```python
from build123d import *

# Parameters (mm, degrees)
BOSS_EXTRUDE1_DEPTH = 7.5
FILLET1_R           = 0.4
SKETCH3_R           = 3
CUT_EXTRUDE2_DEPTH  = 1


with BuildPart() as part:
    # Sketch1 → Boss-Extrude1 (new body)
    with BuildSketch(Plane.XY):
        Polygon((9.332731301, -89.971589642), (0, -80.638858341), (-9.332731301, -89.971589642), align=None)
    extrude(amount=-BOSS_EXTRUDE1_DEPTH)

    # Sketch2 → section 1 of loft1
    with BuildSketch(Plane.XY.offset(1.5875), mode=Mode.PRIVATE) as loft1_s1:
        Polygon((-13.165295331, -91.559089642), (13.165295331, -91.559089642), (0, -78.393794311), align=None)
    # loft from a face of the part (loft1)
    loft([part.faces().sort_by_distance((0, -86.860679209, 0))[0], loft1_s1.sketch])

    # Fillet1
    fillet1_edges = [part.edges().sort_by_distance(p)[0] for p in [
        (-4.666365651, -85.305223992, -7.5),
        (0, -89.971589642, -7.5),
        (4.666365651, -85.305223992, -7.5),
    ]]
    fillet(fillet1_edges, radius=FILLET1_R)

    # Sketch3 → Cut-Extrude2 (cut)
    with BuildSketch(Plane.XY.offset(1.5875)):
        with Locations((0, -86.105845763)):
            Circle(SKETCH3_R)
    extrude(amount=-CUT_EXTRUDE2_DEPTH, mode=Mode.SUBTRACT)


solid = part.part
```
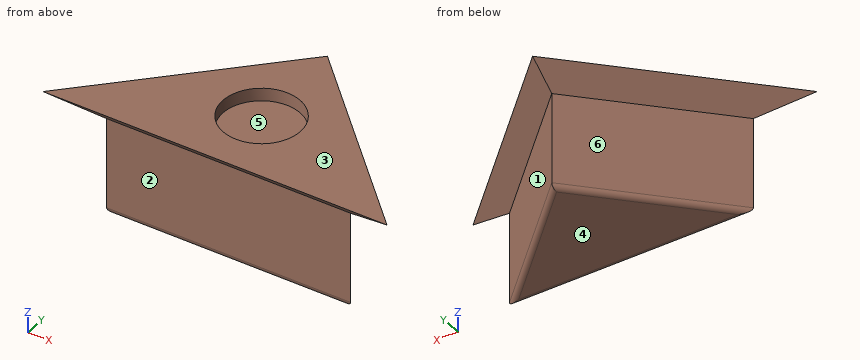
The listing builds one solid part. Answer for the finished solid, in the listing's coordinates (mm). Face numbers are marked on the shaded views. A direction names the side the tool comes from. Coordinates: 2 decimals unless noted, no trailing zeros. Order: outer loops, then holes, each group sorted by start corner. A loop starts at its lowest first (then second) coordinate and runs counter-clockwise, first axis right, second up. Notation, with made-up numbers: M -23.5,-10.75 L 25.5,-10.75 A15 ccw 25.5,4.25 Z; hole C 69.25,89 d1. An arc over 180 degrees is marked long. Answer as a JSON object with one key per item and string values. Group by question number.
1. Section A-A on z = -1 is taken. Write down the section's boundary in (x, y).
2. Flat-ended cylindrical pins translate along their axes: P1, Ø1.5, axis at x = -10.5, z = 0.5, coming from the -Y side; P2, Ø1, axis at x = -2, z = -6, coming from the -Y side; P3, Ø2, axis at y = -80.5, z = -3.5, coming from the +X side. Find the tip coordinate at first contact, or state that the pin passes through.
3. Straight lines are drawn through the part: line 1 (Z direction, x = 0.5, y = -87.5); line 2 (Y direction, x = 1, z = 1); line 3 (Y direction, x = 0.5, z = -2.5). For each, find the intervals that lie inside material, in ascending order.
4. A tool of negligible diameter and unlimited length cuts with its end or side. For the marked faces 1, 2 and 3, from which of +Z, -Z, +X, -X, +Y, -Y can it reach the whole face along a straight path? Write none if from no direction.
5. Determine the mould class of the marked faces 4, 5 and 6 for opening direction X: released by +X, released by -X, zero draft, split by the parting line, or undercut.
Values follow:
{
 "1": {"outline": "M -9.33,-89.97 L 9.33,-89.97 L 0,-80.64 Z"},
 "2": {"P1": "y = -91.22", "P2": "y = -89.97", "P3": "x = 0.86"},
 "3": {"line 1": "-7.5 to 0.59", "line 2": "-90.97 to -88.93, -83.28 to -80.22", "line 3": "-89.97 to -81.14"},
 "4": {"face 1": "-Z, +X, +Y", "face 2": "-Z, +X, -X, -Y", "face 3": "+Z, +X, -X, +Y, -Y"},
 "5": {"face 4": "zero draft", "face 5": "undercut", "face 6": "released by -X"}
}
